```python
from build123d import *

# Parameters (mm, degrees)
F0_W   = 21.5
F0_H   = 4
F0_W_2 = 13.5
F0_W_3 = 3.492
F0_H_2 = 25.2048466533


# Not quite as in the source:
# - a feature names something its author has since deleted; it is built from what else it names


with BuildPart() as f1:
    # F0 (on Front) → F1 (revolve)
    with BuildSketch(Plane.XZ):
        with Locations((-59.25, -12.4232914925)):
            Rectangle(F0_W, F0_H)
        with Locations((-41.75, -12.4232914925)):
            Rectangle(F0_W_2, F0_H)
        with Locations((-71.746, 2.1791318342)):
            Rectangle(F0_W_3, F0_H_2)
        Polygon((-78, -14.4232914925), (-70, -14.4232914925), (-70, -10.4232914925), (-73.492, -10.4232914925), (-74, -10.4232914925), (-78, -10.4232914925), align=None)
    revolve(axis=Axis((-35, 0, -12.4232914925), (0, 0, 1)))


solid = f1.part
```
Input: part model. Units: mm. Frame: model coordinates. A direction names the side the tool comes from. Coordinates: 2 decimals unless noted, no trailing zeros. Write each loop counter-clockwise with the first axis right and the second up, starting at its lowest first coordinate (ties: lowest second). Pieces come first, ordered by that corner, then holes.
1) Section B-B on z = -2. Output: boundary loops of the cut face in (x, y), and give its area (3 significant figures).
2) Set-up query: faces 4 (the flat face through (-35, 0, -10.423)), 5 (the flat face through (-26, 34, 14.782)). Return all of +Z, -Z, +X, -X, +Y, -Y with unobstructed straight access to the full face (end or side cutting, diameter ignored); none if empty.
3) Pin query (flat end, axial travel): pin 1 Ø12 at (x, z) = (-51, 4.5) entering from +Y; pin 2 Ø10 at (y, z) = (-15.5, -4.5) entering from -X; pin 3 Ø3 at (y, z) = (-33.5, 7.5) entering from +X. Return the tip coordinate at first contact, or that it passes through.
4) Mould query, pull axis Y, two halves, no side actions, for faces 1 (the cylindrical face through (-70.56, 14.74, 2.36)), 2 (the flat face through (-67, 22, -10.423)), 3 (the cylindrical face through (-7, 21, 2)). Classes: pulls with the +Y half, pulls with the -Y half, needs draft (parallel to the pull), parting line crosses it, or undercut.
5) Material intervals for line 1 along Y through (x, z) = (-35, 9); line 2 along X through (y, z) = (0, -3.5); line 3 along Z through (x, y) = (-65, -1.5), sorted ascending.
6) Section A-A on y = 0. Output: boundary loops of the cut face in (x, z).
7) Section C-C on x = -35. Output: boundary loops of the cut face in (y, z).
Check result:
1. outline: circle Ø76.98 at (-35, 0); hole circle Ø70 at (-35, 0)
1. area: 806 mm2
2. face 4: +Z
2. face 5: +Z, +X, -X, +Y, -Y
3. pin 1: stops at y = 37.17
3. pin 2: stops at x = -72.03
3. pin 3: stops at x = -13.61
4. face 1: parting line crosses it
4. face 2: needs draft
4. face 3: undercut
5. line 1: y = -38.49 to -35, 35 to 38.49
5. line 2: x = -73.49 to -70, 0 to 3.49
5. line 3: z = -14.42 to -10.42
6. outline: (-78, -14.42) - (8, -14.42) - (8, -10.42) - (3.49, -10.42) - (3.49, 14.78) - (0, 14.78) - (0, -10.42) - (-70, -10.42) - (-70, 14.78) - (-73.49, 14.78) - (-73.49, -10.42) - (-78, -10.42) - close
7. outline: (-43, -14.42) - (43, -14.42) - (43, -10.42) - (38.49, -10.42) - (38.49, 14.78) - (35, 14.78) - (35, -10.42) - (-35, -10.42) - (-35, 14.78) - (-38.49, 14.78) - (-38.49, -10.42) - (-43, -10.42) - close
